Geometry: final body of the model. Coordinates: model frame, mm. Face numbers are marked on the shaded views. A direction names the side the tool comes from. Coordinates: 2 decimals unless noted, no trailing zeros. Order: outer loops, then holes, each group sorted by start corner. A loop starts at its lowest first (then second) coordinate and runs counter-clockwise, first axis right, second up. Notation, with made-up numbers: (8, -7.75) -> (21, -7.75) arc R7 cw to (21, 3.25) -> close; hole circle Ø1 at (38.5, 35.25). An arc over 180 degrees is marked (long way). Answer in a Markdown table with one row per item. Add a question column.
1) Section query B-B on y = 0. Return the cut outline in (x, z), then the cut area to 4 significant figures.
2) Section query C-C on z = 14. Return the cut outline in (x, y).
3) Pull-direction query (Y, two-part tool) for the marked faces 1, 2 and 3; classes: +Y half, -Y half, draft (parallel to the pull), parting line (faces both ways), or undercut.
4) Section query D-D on y = 27.5. Return the cut outline in (x, z), then the cut area to 3 significant figures.
5) Section query A-A on z = 3.75. Return the cut outline in (x, y).
6) Contact query for flat-ended pins moving along their axis: P1, Ø4, axis at x = -1.5, z = 2, coming from the -Y side; P2, Ø5, axis at x = -13.42, y = -7.75, coming from the +Z side; P3, Ø1.5, axis at x = -21.5, z = 12, coming from the -Y side; P4, Ø8, axis at y = -27.5, z = 5.5, coming from the -X side. Output: stop coordinate, or through.
7) Ray query, line 1 (Y direction, x = 0, z = 3.6); line 2 (Y direction, x = 0, z = 22.55); line 3 (Y direction, x = 27.5, z = 22.65). Return the intervals inside material, ascending. Write a range as from..to.
8) Set-up query: the marked faces 4 and 5. Return all of +Z, -Z, +X, -X, +Y, -Y with unobstructed straight access to the full face (end or side cutting, diameter ignored); none if empty.
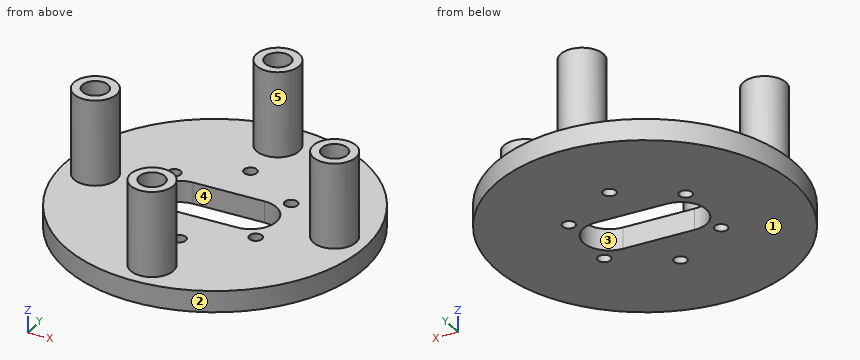
```python
from build123d import *

# Parameters (mm, degrees)
ESBO_O1_R                = 35
RESSALTO_EXTRUS_O1_DEPTH = 5
ESBO_O2_R                = 5
RESSALTO_EXTRUS_O2_DEPTH = 20
ESBO_O3_R                = 3
CORTE_EXTRUS_O1_DEPTH    = 5
CORTE_EXTRUS_O2_DEPTH    = 14
ESBO_O5_R                = 1.5
CORTE_EXTRUS_O3_DEPTH    = 14


with BuildPart() as part:
    # Esboço1 → Ressalto-extrusão1 (new body)
    with BuildSketch(Plane.XY):
        Circle(ESBO_O1_R)
    extrude(amount=RESSALTO_EXTRUS_O1_DEPTH)

    # Esboço2 → Ressalto-extrusão2 (add)
    with BuildSketch(Plane.XY.offset(5)):
        with Locations((27.5, 0)):
            Circle(ESBO_O2_R)
        with Locations((0, -27.5)):
            Circle(ESBO_O2_R)
        with Locations((0, 27.5)):
            Circle(ESBO_O2_R)
        with Locations((-27.5, 0)):
            Circle(ESBO_O2_R)
    extrude(amount=RESSALTO_EXTRUS_O2_DEPTH)

    # Esboço3 → Corte-extrusão1 (cut)
    with BuildSketch(Plane.XY.offset(25)):
        with Locations((0, 27.5)):
            Circle(ESBO_O3_R)
        with Locations((27.5, 0)):
            Circle(ESBO_O3_R)
        with Locations((0, -27.5)):
            Circle(ESBO_O3_R)
        with Locations((-27.5, 0)):
            Circle(ESBO_O3_R)
    extrude(amount=-CORTE_EXTRUS_O1_DEPTH, mode=Mode.SUBTRACT)

    # Esboço4 → Corte-extrusão2 (cut)
    with BuildSketch(Plane.XY.offset(5)):
        with BuildLine():
            Line((8.25, 6), (-8.25, 6))
            ThreePointArc((-8.25, 6), (-14.25, 0), (-8.25, -6))
            Line((-8.25, -6), (8.25, -6))
            ThreePointArc((8.25, -6), (14.25, 0), (8.25, 6))
        make_face()
    extrude(amount=-CORTE_EXTRUS_O2_DEPTH, mode=Mode.SUBTRACT)

    # Esboço5 → Corte-extrusão3 (cut)
    with BuildSketch(Plane.XY.offset(5)):
        with Locations((13.423393759, 7.75)):
            Circle(ESBO_O5_R)
        with Locations((13.423393759, -7.75)):
            Circle(ESBO_O5_R)
        with Locations((0, -15.5)):
            Circle(ESBO_O5_R)
        with Locations((-13.423393759, -7.75)):
            Circle(ESBO_O5_R)
        with Locations((-13.423393759, 7.75)):
            Circle(ESBO_O5_R)
        with Locations((0, 15.5)):
            Circle(ESBO_O5_R)
    extrude(amount=-CORTE_EXTRUS_O3_DEPTH, mode=Mode.SUBTRACT)


solid = part.part
```
Result:
| question | item | result |
|---|---|---|
| 1 | outline | (-35, 0) -> (-14.25, 0) -> (-14.25, 5) -> (-22.5, 5) -> (-22.5, 25) -> (-24.5, 25) -> (-24.5, 20) -> (-30.5, 20) -> (-30.5, 25) -> (-32.5, 25) -> (-32.5, 5) -> (-35, 5) -> close; (14.25, 0) -> (35, 0) -> (35, 5) -> (32.5, 5) -> (32.5, 25) -> (30.5, 25) -> (30.5, 20) -> (24.5, 20) -> (24.5, 25) -> (22.5, 25) -> (22.5, 5) -> (14.25, 5) -> close |
| 1 | area | 547.5 mm2 |
| 2 | outline | circle Ø10 at (-27.5, 0); circle Ø10 at (0, -27.5); circle Ø10 at (0, 27.5); circle Ø10 at (27.5, 0) |
| 3 | face 1 | draft |
| 3 | face 2 | parting line |
| 3 | face 3 | undercut |
| 4 | outline | (-21.65, 0) -> (21.65, 0) -> (21.65, 5) -> (5, 5) -> (5, 25) -> (3, 25) -> (3, 20) -> (-3, 20) -> (-3, 25) -> (-5, 25) -> (-5, 5) -> (-21.65, 5) -> close |
| 4 | area | 387 mm2 |
| 5 | outline | circle Ø70 at (0, 0); hole circle Ø3 at (-13.42, -7.75); hole circle Ø3 at (-13.42, 7.75); hole (-8.25, -6) -> (8.25, -6) arc R6 ccw to (8.25, 6) -> (-8.25, 6) arc R6 ccw to start; hole circle Ø3 at (0, -15.5); hole circle Ø3 at (0, 15.5); hole circle Ø3 at (13.42, -7.75); hole circle Ø3 at (13.42, 7.75) |
| 6 | P1 | y = -35 |
| 6 | P2 | z = 5 |
| 6 | P3 | through |
| 6 | P4 | x = -25.91 |
| 7 | line 1 | -35..-17, -14..-6, 6..14, 17..35 |
| 7 | line 2 | -32.5..-30.5, -24.5..-22.5, 22.5..24.5, 30.5..32.5 |
| 7 | line 3 | -5..-3, 3..5 |
| 8 | face 4 | +Z, -Z |
| 8 | face 5 | +Z |
